```python
from build123d import *

# Parameters (mm, degrees)
SKETCH1_W           = 190.5
SKETCH1_H           = 25.4
SKETCH1_R           = 2.4892
SKETCH1_W_2         = 50.8
SKETCH1_H_2         = 50.8
BOSS_EXTRUDE1_DEPTH = 3.175
FILLET1_R           = 4.7625


with BuildPart() as part:
    # Sketch1 → Boss-Extrude1 (new body)
    with BuildSketch(Plane(origin=(0, 0, 0), x_dir=(1, 0, 0), z_dir=(0, 1, 0))):
        with Locations((95.25, 12.7)):
            Rectangle(SKETCH1_W, SKETCH1_H)
        with Locations((6.35, 12.7)):
            Circle(SKETCH1_R, mode=Mode.SUBTRACT)
        with Locations((31.75, 12.7)):
            Circle(SKETCH1_R, mode=Mode.SUBTRACT)
        with Locations((57.15, 12.7)):
            Circle(SKETCH1_R, mode=Mode.SUBTRACT)
        with Locations((82.55, 12.7)):
            Circle(SKETCH1_R, mode=Mode.SUBTRACT)
        with Locations((107.95, 12.7)):
            Circle(SKETCH1_R, mode=Mode.SUBTRACT)
        with Locations((133.35, 12.7)):
            Circle(SKETCH1_R, mode=Mode.SUBTRACT)
        with Locations((158.75, 12.7)):
            Circle(SKETCH1_R, mode=Mode.SUBTRACT)
        with Locations((184.15, 12.7)):
            Circle(SKETCH1_R, mode=Mode.SUBTRACT)
        with Locations((95.25, -25.4)):
            Rectangle(SKETCH1_W_2, SKETCH1_H_2)
        with Locations((82.55, -6.35)):
            Circle(SKETCH1_R, mode=Mode.SUBTRACT)
        with Locations((107.95, -6.35)):
            Circle(SKETCH1_R, mode=Mode.SUBTRACT)
        with Locations((107.95, -25.4)):
            Circle(SKETCH1_R, mode=Mode.SUBTRACT)
        with Locations((107.95, -44.45)):
            Circle(SKETCH1_R, mode=Mode.SUBTRACT)
        with Locations((82.55, -25.4)):
            Circle(SKETCH1_R, mode=Mode.SUBTRACT)
        with Locations((82.55, -44.45)):
            Circle(SKETCH1_R, mode=Mode.SUBTRACT)
    extrude(amount=BOSS_EXTRUDE1_DEPTH)

    # Fillet1
    fillet1_edges = [part.edges().sort_by_distance(p)[0] for p in [
        (120.65, 1.5875, 50.8),
        (69.85, 1.5875, 50.8),
        (69.85, 1.5875, 0),
        (0, 1.5875, 0),
        (0, 1.5875, -25.4),
        (190.5, 1.5875, -25.4),
        (190.5, 1.5875, 0),
        (120.65, 1.5875, 0),
    ]]
    fillet(fillet1_edges, radius=FILLET1_R)


solid = part.part
```
The listing builds one solid part. Answer for the finished solid, in the listing's coordinates (mm). A direction names the side the tool comes from. Coordinates: 2 decimals unless noted, no trailing zeros. Write each loop counter-clockwise with the first axis right and the second up, starting at its lowest first coordinate (ties: lowest second). Pieces come first, ordered by that corner, then holes. Notation, with made-up numbers: (-19, -3.5) - (23, -3.5) arc R21 cw to (23, 29.5) - close; hole circle Ø1 at (-24.75, 73). An arc over 180 degrees is marked (long way). One line per item, written item: value.
1) Consider line 1 along Z through (x, y) = (82.55, 2.3); line 2 along X through (y, z) = (1.2, 6.35); line 3 along X through (y, z) = (1.4, 43.5). Determine where each line is inside the solid, lowest interval first. Write a range as from..to.
Geometry check:
line 1: z = -25.4..-15.19, -10.21..3.86, 8.84..22.91, 27.89..41.96, 46.94..50.8
line 2: x = 69.85..80.06, 85.04..105.46, 110.44..120.65
line 3: x = 69.85..80.25, 84.85..105.65, 110.25..120.65
2) A tool of negligible diameter and unlimited length cuts with its end or side. For faces 5 (the flat face through (155, 2, 0)), 6 (the cylindrical face through (1.36, 1.61, -1.43)), from which of +Z, -Z, +X, -X, +Y, -Y can it reach the whole face along a straight path? Write none if from no direction.
Geometry check:
face 5: +Z, +X, +Y, -Y
face 6: +Z, -X, +Y, -Y
3) Each of these flat-tipped pins is pushed along its axis until it touches: pin 1 Ø1.6 at (y, z) = (2, 15) entering from +X; pin 2 Ø1 at (x, y) = (47.5, 1.5) entering from +Z; pin 3 Ø1 at (y, z) = (0.5, 29.5) entering from -X. Where does it stop, or does it pass through?
Geometry check:
pin 1: stops at x = 120.65
pin 2: stops at z = 0
pin 3: stops at x = 69.85
4) Find section B-B (y = 0.5). Count the separate pieces of the cut face and the enclosed holes in it, and give its area (3 significant figures).
Geometry check:
separate pieces: 1
enclosed holes: 14
area: 7,130 mm2
5) Find section A-A (z = 25.4). Give the vertices of the cut face in (x, y) (3 decimals).
Geometry check:
outline: (69.85, 0) - (80.061, 0) - (80.061, 3.175) - (69.85, 3.175) - close; (85.039, 0) - (105.461, 0) - (105.461, 3.175) - (85.039, 3.175) - close; (110.439, 0) - (120.65, 0) - (120.65, 3.175) - (110.439, 3.175) - close
6) Find section C-C (x = 31.75). Give the vertices of the cut face in (y, z) (3 decimals), and give its area (3 significant figures).
Geometry check:
outline: (0, -25.4) - (3.175, -25.4) - (3.175, -15.189) - (0, -15.189) - close; (0, -10.211) - (3.175, -10.211) - (3.175, 0) - (0, 0) - close
area: 64.8 mm2
7) Find section D-D (x = 174). Give the vertices of the cut face in (y, z) (3 decimals).
Geometry check:
outline: (0, -25.4) - (3.175, -25.4) - (3.175, 0) - (0, 0) - close
8) For a pull along X with two mould halves and no side action, classify faces 1 (the flat face through (0, 2, -13)), 2 (the cylindrical face through (189.07, 1.61, -24.04)), 3 (the cylindrical face through (161.124, 1.565, -13.448)), 4 (the cylindrical face through (105.463, 1.565, -12.809)) as pulls with the +X half, pulls with the -X half, needs draft (parallel to the pull), parting line crosses it, or undercut.
Geometry check:
face 1: pulls with the -X half
face 2: pulls with the +X half
face 3: undercut
face 4: undercut
